from build123d import *

# Parameters (mm, degrees)
SKETCH_1_R          = 2
EXTRUDE_1_DEPTH     = 40
SKETCH_2_R          = 3.515
EXTRUDE_2_DEPTH     = 3
CUT_EXTRUDE_1_DEPTH = 1
CUT_EXTRUDE_1_DRAFT = -12
FILLET_2_R          = 1


with BuildPart() as part:
    # Эскиз1 → Бобышка-Вытянуть1 (new body)
    with BuildSketch(Plane(origin=(0, 0, 0), x_dir=(1, 0, 0), z_dir=(0, 1, 0))):
        with Locations(Location((0, 0, 0), (0, 0, 270))):
            Circle(SKETCH_1_R)
    extrude(amount=EXTRUDE_1_DEPTH)

    # Эскиз2 → Бобышка-Вытянуть2 (add)
    with BuildSketch(Plane(origin=(0, 40, 0), x_dir=(1, 0, 0), z_dir=(0, 1, 0))):
        with Locations(Location((0, 0, 0), (0, 0, 270))):
            Circle(SKETCH_2_R)
    extrude(amount=EXTRUDE_2_DEPTH)


with BuildPart() as cut_extrude_1_tool:
    # Эскиз3 → Вырез-Вытянуть1 (with draft: the straight prism first)
    with BuildSketch(Plane(origin=(0, 43, 0), x_dir=(1, 0, 0), z_dir=(0, 1, 0))):
        Polygon((-2.641549473, 0.422769916), (-2.641549473, -0.422769916), (-0.422769916, -0.422769916), (-0.422769916, -2.641549473), (0.422769916, -2.641549473), (0.422769916, -0.422769916), (2.641549473, -0.422769916), (2.641549473, 0.422769916), (0.422769916, 0.422769916), (0.422769916, 2.641549473), (-0.422769916, 2.641549473), (-0.422769916, 0.422769916), align=None)
    extrude(amount=-CUT_EXTRUDE_1_DEPTH)
    # Вырез-Вытянуть1: the draft: its side faces are tilted about the plane it starts from
    cut_extrude_1_sides = [cut_extrude_1_tool.faces().sort_by_distance(p)[0] for p in [
        (-2.641549473, 42.5, 0),
        (-1.532159694, 42.5, 0.422769916),
        (-0.422769916, 42.5, 1.532159694),
        (0, 42.5, 2.641549473),
        (0.422769916, 42.5, 1.532159694),
        (1.532159694, 42.5, 0.422769916),
        (2.641549473, 42.5, 0),
        (1.532159694, 42.5, -0.422769916),
        (0.422769916, 42.5, -1.532159694),
        (0, 42.5, -2.641549473),
        (-0.422769916, 42.5, -1.532159694),
        (-1.532159694, 42.5, -0.422769916),
    ]]
    draft(cut_extrude_1_sides, Plane(origin=(0, 43, 0), x_dir=(1, 0, 0), z_dir=(0, 1, 0)), CUT_EXTRUDE_1_DRAFT)


with BuildPart() as part_1:
    add(part.part)

    # Вырез-Вытянуть1: cut by cut_extrude_1_tool
    add(cut_extrude_1_tool.part, mode=Mode.SUBTRACT)

    # Скругление2
    # the kernel refuses this fillet: 1 mm, written as the material it takes off along each edge
    with BuildSketch(Plane(origin=(0, 43, 0), x_dir=(0, 0, 1), z_dir=(-1, 0, 0))) as fillet_2_piece_1:
        with BuildLine():
            CenterArc((3.515 - FILLET_2_R, -FILLET_2_R), FILLET_2_R, 0, 90)
            Line((3.515 - FILLET_2_R, 0), (3.515, 0))
            Line((3.515, 0), (3.515, -FILLET_2_R))
        make_face()
    revolve(axis=Axis((0, 43, 0), (0, 1, 0)), mode=Mode.SUBTRACT)


solid = part_1.part
Here's how the part is built. I have some questions about the finished solid (model axes, mm). A direction names the side the tool comes from. Round coordinates to 2 decimals unless told otherwise and drop trailing zeros. Order: outer loops, then holes, each group sorted by start corner. A loop starts at its lowest first (then second) coordinate and runs counter-clockwise, first axis right, second up. Notation, with made-up numbers: (1.5, 85) -> (28.5, 85) arc R27 ccw to (28.5, 119) -> close; hole circle Ø10 at (57, -38). An arc over 180 degrees is marked (long way). Use CSV: the item, a comma, the result in double quotes.
1. Which directions (+Z, -Z, +X, -X, +Y, -Y) give clear straight access to the entire face, cutting with the end or side of a thin tool? Please do faces 1 (the face through (1, 43, 1)), 2 (the face through (-2, 40, 2)), 3 (the face through (1.41, 42.51, 0.32)).
Recorded:
face 1,"+Z, -Z, +X, -X, +Y"
face 2,"-Y"
face 3,"+Y"
2. I need wall thicknesses on line 1 along Y through (x, z) = (-2.5, 0.75); line 2 along Y through (x, z) = (0, 0); line 3 along X through (y, z) = (9.5, 1.75). Which ranges of each line are inside material? Lowest first, please.
Recorded:
line 1,"y = 40 to 43"
line 2,"y = 0 to 42"
line 3,"x = -0.97 to 0.97"
3. Thinking about a two-plate mould opening in X: for faces 4 (the face through (-2, 20, 0)), 5 (the face through (1, 43, -1)), 6 (the face through (-1.41, 42.51, -0.32)), which applies, pulls with the +X half, pulls with the -X half, needs draft (parallel to the pull), parting line crosses it, or undercut?
Recorded:
face 4,"parting line crosses it"
face 5,"needs draft"
face 6,"undercut"
4. I want a section at A-A on y = 9.5. List the corners of the cut face in (x, z) for me, and give its area (3 significant figures).
Recorded:
outline,"circle Ø4 at (0, 0)"
area,"12.6 mm2"
5. I'm going to push flat-ended pins straight in: P1, Ø1.5, axis at x = 0.5, y = 33, coming from the -Z side; P2, Ø1.5, axis at y = 26.5, z = 2.5, coming from the +X side; P3, Ø3, axis at y = 25.5, z = 1.5, coming from the -X side. Where does each tip first touch, or does it pass through?
Recorded:
P1,"stops at z = -2"
P2,"stops at x = 0.97"
P3,"stops at x = -2"
